The model under review builds one solid part; all positions refer to its coordinate system, in mm. Face numbers are marked on the shaded views. A direction names the side the tool comes from. Give positions to 0.01 mm unless a question says otherwise; leave off trailing zeros. Write each loop counter-clockwise with the first axis right and the second up, starting at its lowest first coordinate (ties: lowest second). Pieces come first, ordered by that corner, then holes. Notation, with made-up numbers: M 35.5,38.5 L 85.5,38.5 A20 cw 85.5,62.5 Z; hole C 66,13.25 d2. An arc over 180 degrees is marked long. Write item = value, one per line. Start each with the question number.
Autodesk Inventor part; units mm, degrees
ref_plane "YZ Plane" through (0, 0, 0) normal (1, 0, 0) x (0, 1, 0)
ref_plane "XZ Plane" through (0, 0, 0) normal (0, 1, 0) x (-1, 0, 0)
ref_plane "XY Plane" through (0, 0, 0) normal (0, 0, 1) x (1, 0, 0)
sketch "Sketch1" plane through (0, 0, 0) normal (0, 0, 1) x (1, 0, 0)
  circle A0 centre (34.0048, -4) radius 3.4
  line L0 (31.935, 7.7219) -> (31.935, 3.2459)
  arc A1 (32.564, 8.35) -> (31.935, 7.7219) centre (32.5699, 7.7151) ccw
  line L1 (35.5549, 8.35) -> (32.564, 8.35)
  arc A2 (38.35, 5.4968) -> (35.5549, 8.35) centre (35.557, 5.5563) ccw
  line L2 (38.35, 2.5356) -> (38.35, 5.4968)
  arc A3 (37.6808, 1.976) -> (38.35, 2.5356) centre (37.7194, 2.6098) ccw
  line L3 (33.2048, 1.976) -> (37.6808, 1.976)
  arc A4 (31.935, 3.2459) -> (33.2048, 1.976) centre (33.2048, 3.2459) ccw
  line L4 (-13.4502, -6.9544) -> (13.4502, -6.9544)
  arc A5 (-13.8991, -5.8705) -> (-13.4502, -6.9544) centre (-13.4502, -6.3195) ccw
  line L5 (-1.2578, 6.7693) -> (-13.8991, -5.8705)
  arc A6 (-0.8088, 6.9553) -> (-1.2578, 6.7693) centre (-0.8088, 6.3203) ccw
  line L6 (0.8088, 6.9553) -> (-0.8088, 6.9553)
  arc A7 (1.2578, 6.7693) -> (0.8088, 6.9553) centre (0.8088, 6.3203) ccw
  line L7 (13.8991, -5.8705) -> (1.2578, 6.7693)
  arc A8 (13.4502, -6.9544) -> (13.8991, -5.8705) centre (13.4502, -6.3195) ccw
  line L8 (-37.7151, 1.9604) -> (-33.2048, 1.9604)
  arc A9 (-38.35, 2.5953) -> (-37.7151, 1.9604) centre (-37.7151, 2.5953) ccw
  line L9 (-38.35, 5.5571) -> (-38.35, 2.5953)
  arc A10 (-35.4935, 8.35) -> (-38.35, 5.5571) centre (-35.5563, 5.5571) ccw
  line L10 (-32.5699, 8.35) -> (-35.4935, 8.35)
  arc A11 (-31.935, 7.7151) -> (-32.5699, 8.35) centre (-32.5699, 7.7151) ccw
  line L11 (-31.935, 3.2302) -> (-31.935, 7.7151)
  arc A12 (-33.2048, 1.9604) -> (-31.935, 3.2302) centre (-33.2048, 3.2302) ccw
  circle A13 centre (-34.0048, -4) radius 3.4
  line L12 (13.2285, 5.9365) -> (14.3654, 5.9365)
  arc A14 (14.3654, 5.9365) -> (15.94, 7.5111) centre (14.3654, 7.5111) ccw
  line L13 (15.94, 7.5111) -> (15.94, 8.4254)
  arc A15 (15.94, 8.4254) -> (14.5525, 10) centre (14.3654, 8.4365) ccw
  line L14 (14.5525, 10) -> (-14.3654, 10)
  arc A16 (-14.3654, 10) -> (-15.94, 8.4254) centre (-14.3654, 8.4254) ccw
  line L15 (-15.94, 8.4254) -> (-15.94, 7.5111)
  arc A17 (-15.94, 7.5111) -> (-14.3654, 5.9365) centre (-14.3654, 7.5111) ccw
  line L16 (-14.3654, 5.9365) -> (-13.2285, 5.9365)
  line L17 (-13.2285, 5.9365) -> (-13.2285, 6.4054)
  line L18 (-13.2285, 6.4054) -> (-10.9848, 6.4054)
  arc A18 (-9.715, 5.1355) -> (-10.9848, 6.4054) centre (-10.9848, 5.1355) ccw
  line L19 (-9.715, 5.1355) -> (-9.715, 2.6208)
  arc A19 (-9.9753, 1.9923) -> (-9.715, 2.6208) centre (-10.6039, 2.6208) ccw
  line L20 (-9.9753, 1.9923) -> (-12.8764, -0.9089)
  arc A20 (-16.2347, -2.3) -> (-12.8764, -0.9089) centre (-16.2347, 2.4492) ccw
  line L21 (-16.2347, -2.3) -> (-23.5072, -2.3)
  arc A21 (-26.8655, -0.9089) -> (-23.5072, -2.3) centre (-23.5072, 2.4492) ccw
  line L22 (-26.8655, -0.9089) -> (-30.0247, 2.2504)
  arc A22 (-30.285, 2.879) -> (-30.0247, 2.2504) centre (-29.3961, 2.879) ccw
  line L23 (-30.285, 2.879) -> (-30.285, 5.1355)
  arc A23 (-29.0152, 6.4054) -> (-30.285, 5.1355) centre (-29.0152, 5.1355) ccw
  line L24 (-29.0152, 6.4054) -> (-26.8986, 6.4054)
  line L25 (-26.8986, 6.4054) -> (-26.8986, 5.9365)
  line L26 (-26.8986, 5.9365) -> (-25.7617, 5.9365)
  arc A24 (-25.7617, 5.9365) -> (-24.06, 7.506) centre (-25.6346, 7.506) ccw
  line L27 (-24.06, 7.506) -> (-24.06, 8.4203)
  arc A25 (-24.06, 8.4203) -> (-25.7617, 10) centre (-25.6441, 8.4203) ccw
  line L28 (-25.7617, 10) -> (-36.8282, 10)
  arc A26 (-36.8282, 10) -> (-40, 6.8282) centre (-36.8282, 6.8282) ccw
  line L29 (-40, 6.8282) -> (-40, -6.8282)
  arc A27 (-40, -6.8282) -> (-36.8282, -10) centre (-36.8282, -6.8282) ccw
  line L30 (-36.8282, -10) -> (36.8254, -10)
  arc A28 (36.8254, -10) -> (40, -6.8282) centre (36.8254, -6.8254) ccw
  line L31 (40, -6.8282) -> (40, 6.8282)
  arc A29 (40, 6.8282) -> (36.8854, 10) centre (36.8254, 6.826) ccw
  line L32 (36.8854, 10) -> (25.4475, 10)
  arc A30 (25.4475, 10) -> (24.06, 8.4254) centre (25.6346, 8.4365) ccw
  line L33 (24.06, 8.4254) -> (24.06, 7.5111)
  arc A31 (24.06, 7.5111) -> (25.6346, 5.9365) centre (25.6346, 7.5111) ccw
  line L34 (25.6346, 5.9365) -> (26.7715, 5.9365)
  line L35 (26.7715, 5.9365) -> (26.7715, 6.6606)
  line L36 (26.7715, 6.6606) -> (29.0152, 6.6606)
  arc A32 (30.285, 5.3908) -> (29.0152, 6.6606) centre (29.0152, 5.3908) ccw
  line L37 (30.285, 5.3908) -> (30.285, 3.1342)
  arc A33 (30.0247, 2.2504) -> (30.285, 3.1342) centre (29.4256, 2.9071) ccw
  line L38 (30.0247, 2.2504) -> (26.8655, -0.9089)
  arc A34 (23.5072, -2.3) -> (26.8655, -0.9089) centre (23.5072, 2.4492) ccw
  line L39 (23.5072, -2.3) -> (16.4928, -2.3)
  arc A35 (13.1345, -0.6536) -> (16.4928, -2.3) centre (16.7353, 2.443) ccw
  line L40 (13.1345, -0.6536) -> (9.9753, 2.5057)
  arc A36 (9.715, 3.1342) -> (9.9753, 2.5057) centre (10.6039, 3.1342) ccw
  line L41 (9.715, 3.1342) -> (9.715, 5.3908)
  arc A37 (10.9848, 6.6606) -> (9.715, 5.3908) centre (10.9848, 5.3908) ccw
  line L42 (10.9848, 6.6606) -> (13.2285, 6.6606)
  line L43 (13.2285, 6.6606) -> (13.2285, 5.9365)
  point P0 (0, 0)
extrude "Extrusion1" add sketch "Sketch1" against normal blind 100
properties part number "40-8020.dxf"
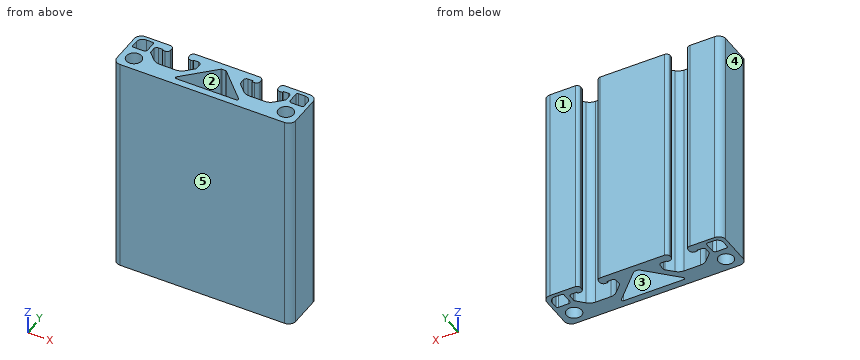
Item 1: Clearance check with a flat-ended pin moving along its axis: P1, Ø7.5, axis at x = 18.5, z = -46.5, coming from the +Y side. State where the tip first meets the part, or that it passes through.
Item 2: For the marked faces 1 and 2, list the 3-axis set-ups (+Z, -Z, +X, -X, +Y, -Y) from which the entire face can be reached by the end or side of a thin tool; tool diameter is ignored.
Item 3: We need section C-C, the plane z = -25.5. Give the number of separate pieces and of enclosed holes in the cut face, and give its area (3 significant figures).
Item 4: The part is to be moulded in two halves that separate along X. For the marked faces 3, 4 and 5, say which applies: released by +X, released by -X, zero draft, split by the parting line, or undercut.
Item 5: To check wall thickness, follow probe 1 along Y at (x, z) = (11.5, -39); probe 2 along X at (y, z) = (9, -65); probe 3 along Y at (x, z) = (34, -69). State the ranges of each line that lie inside material, in increasing order. Write a range as [from, to].
Item 6: We need section B-B, the plane x = 8. Write out the cut boundary in (y, z).
Item 7: We need section D-D, the plane x = -20. Write out the cut boundary in (y, z), and give its area (3 significant figures).
Item 8: We need section A-A, the plane y = -4. Write out the cut boundary in (x, z), and give its area (3 significant figures).
Worked out:
q1.P1 = 9.96
q2.face_1 = +Z, -Z, +X, -X, +Y
q2.face_2 = +Z, -Z
q3.separate_pieces = 1
q3.enclosed_holes = 5
q3.area = 851 mm²
q4.face_3 = undercut
q4.face_4 = released by -X
q4.face_5 = zero draft
q5.probe_1 = [-10, -6.95], [-3.47, 0.98], [6.66, 10]
q5.probe_2 = [-39.14, -24.17], [-15.83, 15.84], [24.16, 39.14]
q5.probe_3 = [-10, -7.4], [-0.6, 1.98], [8.35, 10]
q6.outline = M -10,-100 L -6.95,-100 L -6.95,0 L -10,0 Z; M 0.03,-100 L 10,-100 L 10,0 L 0.03,0 Z
q7.outline = M -10,-100 L -2.3,-100 L -2.3,0 L -10,0 Z
q7.area = 770 mm²
q8.outline = M -40,-100 L -37.4,-100 L -37.4,0 L -40,0 Z; M -30.6,-100 L -12.03,-100 L -12.03,0 L -30.6,0 Z; M 12.03,-100 L 30.6,-100 L 30.6,0 L 12.03,0 Z; M 37.4,-100 L 40,-100 L 40,0 L 37.4,0 Z
q8.area = 4,230 mm²
